from build123d import *

# Parameters (mm, degrees)
F1_DEPTH = 25.4
F3_DEPTH = 25.4


with BuildPart() as f1:
    # F0 (on Front) → F1 (new body)
    with BuildSketch(Plane.XZ):
        Polygon((-199.5275318623, -22.8119939566), (-180.0614446402, -29.4490549713), (-173.5727488995, -41.6347756982), (-196.6436803341, -45.4109199345), (-162.3977720737, -54.6305887401), (-168.5259789228, -17.4674503505), (-150.5018025637, -30.1844198257), (-150.5018025637, 0), (-176.8171042204, 5.3729466163), align=None)
    extrude(amount=F1_DEPTH)

    # F2 (on Front) → F3 (join)
    with BuildSketch(Plane.XZ):
        with BuildLine():
            Line((-109.767191112, 61.2932294607), (-126.709908247, 61.2932294607))
            Line((-126.709908247, 61.2932294607), (-126.709908247, 39.4931892306))
            ThreePointArc((-126.709908247, 39.4931892306), (-117.6753186658, 37.0409814921), (-109.767191112, 32.031126176))
            Line((-109.767191112, 32.031126176), (-109.767191112, 61.2932294607))
        make_face()
        with BuildLine():
            ThreePointArc((-109.767191112, 32.031126176), (-117.6753186658, 37.0409814921), (-126.709908247, 39.4931892306))
            Line((-126.709908247, 39.4931892306), (-126.709908247, 24.0076240152))
            Line((-126.709908247, 24.0076240152), (-109.767191112, 24.0076240152))
            Line((-109.767191112, 24.0076240152), (-109.767191112, 32.031126176))
        make_face()
        with BuildLine():
            Line((-126.709908247, 24.0076240152), (-126.709908247, 39.4931892306))
            ThreePointArc((-126.709908247, 39.4931892306), (-141.5942846277, 37.6022015758), (-153.8963533146, 29.0126963179))
            ThreePointArc((-153.8963533146, 29.0126963179), (-141.3568088034, -21.0066330726), (-98.9566655593, 8.3430064842))
            ThreePointArc((-98.9566655593, 8.3430064842), (-101.7870306722, 21.3621700255), (-109.767191112, 32.031126176))
            Line((-109.767191112, 32.031126176), (-109.767191112, 24.0076240152))
            Line((-109.767191112, 24.0076240152), (-126.709908247, 24.0076240152))
        make_face()
    extrude(amount=F3_DEPTH)


solid = f1.part
For this review, take the finished solid that the model builds, in its own axes (mm). A direction names the side the tool comes from. Coordinates: 2 decimals unless noted, no trailing zeros. Order: outer loops, then holes, each group sorted by start corner. A loop starts at its lowest first (then second) coordinate and runs counter-clockwise, first axis right, second up. Notation, with made-up numbers: (77.5, 59) - (115.5, 59) arc R27 ccw to (115.5, 90) - close; hole circle Ø4 at (75.5, 19.25). An arc over 180 degrees is marked (long way). Use one line per item in the form item = value.
Q1. For P1, Ø2, axis at x = -121.5, z = -15.5, coming from the +Y side; P2, Ø1.5, axis at y = -5, z = 46, coming from the +X side; P3, Ø1, axis at x = -112, y = -14.5, coming from the -Z side, all flat-tipped, find the tip position at first contact; note any pin that passes through.
Checked values:
P1 = 0
P2 = -109.77
P3 = -17.46
Q2. Draft analysis for pull direction X (two halves, no side actions). For faces 4 (the flat face through (-184.947, -12.522, -43.496)), 5 (the flat face through (-109.767, -13, 46)), 6 (the flat face through (-165.42, -12.52, -36.31)), 7 (the flat face through (-118, -13, 61.293)), state which applies: +X half, -X half, draft (parallel to the pull), parting line (faces both ways), or undercut.
Checked values:
face_4 = -X half
face_5 = +X half
face_6 = undercut
face_7 = draft
Q3. Consider section D-D (z = -40). Give the boundary of the cut face in (x, y).
Checked values:
outline = (-174.44, -25.4) - (-164.81, -25.4) - (-164.81, 0) - (-174.44, 0) - close
Q4. Consider section B-B (z = -20). Give the boundary of the cut face in (x, y).
Checked values:
outline = (-197.26, -25.4) - (-168.11, -25.4) - (-168.11, 0) - (-197.26, 0) - close; (-164.94, -25.4) - (-150.5, -25.4) - (-150.5, 0) - (-164.94, 0) - close; (-143.73, -25.4) - (-116.9, -25.4) - (-116.9, 0) - (-143.73, 0) - close
Q5. For probe 1 along Z at (x, y) = (-193, -21.75); probe 2 along Z at (x, y) = (-180, -7.5); probe 3 along Z at (x, y) = (-169, -14.5), list the stretches that pass through material, from the lowest coordinate up. Write a range as from..to.
Checked values:
probe_1 = -46.39..-44.81, -25.04..-14.71
probe_2 = -49.89..-42.69, -29.56..1.42
probe_3 = -52.85..3.78
Q6. For faces 1 (the flat face through (-176.86, -12.52, -35.46)), 2 (the flat face through (-150.502, -13, -23)), 3 (the flat face through (-159.64, -12.522, -23.737)), list the 3-axis set-ups (+Z, -Z, +X, -X, +Y, -Y) from which the entire face can be reached by the end or side of a thin tool; tool diameter is ignored.
Checked values:
face_1 = -X, +Y, -Y
face_2 = -Z, +Y, -Y
face_3 = +Y, -Y
Q7. Consider section C-C (x = -192). Give the boundary of the cut face in (y, z), then the cut area to 3 significant figures.
Checked values:
outline = (-25.4, -46.66) - (0, -46.66) - (0, -44.65) - (-25.4, -44.65) - close; (-25.4, -25.38) - (0, -25.38) - (0, -13.47) - (-25.4, -13.47) - close
area = 354 mm2
